Can you work these out from the model? Positions are in its coordinate system, mm. Face numbers are marked on the shaded views. A direction names the side the tool comes from. Give positions to 0.01 mm unless a question says otherwise; leave off trailing zeros. Order: outer loops, then holes, each group sorted by start corner. A loop starts at its lowest first (then second) coordinate and runs counter-clockwise, first axis right, second up. Notation, with made-up numbers: (63, 3.5) - (87, 3.5) arc R19 cw to (87, 7.5) - close; hole circle Ø11 at (30, -6.75). An arc over 180 degrees is marked (long way). Return JSON: item names as keys, results as strings.
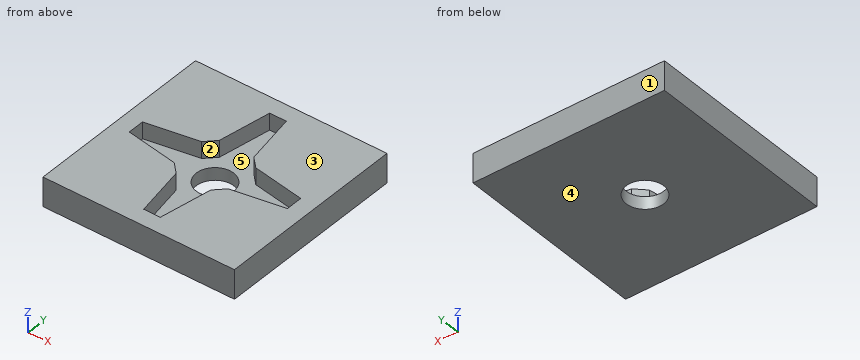
```python
from build123d import *

# Parameters (mm, degrees)
SKETCH1_W           = 46
SKETCH1_H           = 46
BOSS_EXTRUDE1_DEPTH = 7
SKETCH2_W           = 46
SKETCH2_H           = 46
BOSS_EXTRUDE2_DEPTH = 3
SKETCH3_R           = 4.5
CUT_EXTRUDE1_DEPTH  = 3
CUT_EXTRUDE2_DEPTH  = 4


with BuildPart() as part:
    # Sketch1 → Boss-Extrude1 (new body)
    with BuildSketch(Plane.XY):
        Rectangle(SKETCH1_W, SKETCH1_H)
        Polygon((-2, 19), (2, 19), (4.5, 4.5), (19, 2), (19, -2), (4.5, -4.5), (2, -19), (-2, -19), (-4.5, -4.5), (-19, -2), (-19, 2), (-4.5, 4.5), align=None, mode=Mode.SUBTRACT)
    extrude(amount=BOSS_EXTRUDE1_DEPTH)

    # Sketch2 → Boss-Extrude2 (add)
    with BuildSketch(Plane.XY):
        Rectangle(SKETCH2_W, SKETCH2_H)
    extrude(amount=BOSS_EXTRUDE2_DEPTH)

    # Sketch3 → Cut-Extrude1 (cut)
    with BuildSketch(Plane.XY):
        Circle(SKETCH3_R)
    extrude(amount=CUT_EXTRUDE1_DEPTH, mode=Mode.SUBTRACT)

    # Sketch4 → Cut-Extrude2 (cut)
    with BuildSketch(Plane.XY.offset(7)):
        Polygon((-4.155172414, 6.5), (-6.5, 4.155172414), (-6.5, -4.155172414), (-4.155172414, -6.5), (4.155172414, -6.5), (6.5, -4.155172414), (6.5, 4.155172414), (4.155172414, 6.5), align=None)
    extrude(amount=-CUT_EXTRUDE2_DEPTH, mode=Mode.SUBTRACT)


solid = part.part
```
1. Thinking about a two-plate mould opening in Y: for the marked faces 1, 2 and 3, which applies, +Y half, -Y half, draft (parallel to the pull), parting line (faces both ways), or undercut?
Checks:
{"face 1": "+Y half", "face 2": "undercut", "face 3": "draft"}
2. Suppose I cut it at D-D (y = 11). List the corners of the cut face in (x, z) for me.
Checks:
{"outline": "(-23, 0) - (23, 0) - (23, 7) - (3.38, 7) - (3.38, 3) - (-3.38, 3) - (-3.38, 7) - (-23, 7) - close"}
3. On a 3-axis mill with a long thin cutter (end or side, diameter ignored), from which of +Z, -Z, +X, -X, +Y, -Y can I reach the whole of each face in a straight line? I mean the marked faces 4 and 5. Say none if no direction works.
Checks:
{"face 4": "-Z, +X, -X, +Y, -Y", "face 5": "+Z"}
4. If I drill on L1, parallel to Y at x = 0, z = 1.15; L2, parallel to Y at x = -1.5, z = 6.25; L3, parallel to Z at x = -6.5, y = 3, over which ranges is the centre line in solid material (lowest first)? Write a range as [from, to].
Checks:
{"L1": "[-23, -4.5], [4.5, 23]", "L2": "[-23, -19], [19, 23]", "L3": "[0, 3]"}
5. Suppose I cut it at A-A (z = 6.25). List the corners of the cut face in (x, y) for me, plus the area to 3 significant figures.
Checks:
{"outline": "(-23, -23) - (23, -23) - (23, 23) - (-23, 23) - close; hole (-19, -2) - (-6.5, -4.16) - (-4.16, -6.5) - (-2, -19) - (2, -19) - (4.16, -6.5) - (6.5, -4.16) - (19, -2) - (19, 2) - (6.5, 4.16) - (4.16, 6.5) - (2, 19) - (-2, 19) - (-4.16, 6.5) - (-6.5, 4.16) - (-19, 2) - close", "area": "1,650 mm^2"}
6. Suppose I cut it at B-B (y = 0). List the corners of the cut face in (x, z) for me, plus the area to 3 significant figures.
Checks:
{"outline": "(-23, 0) - (-4.5, 0) - (-4.5, 3) - (-19, 3) - (-19, 7) - (-23, 7) - close; (4.5, 0) - (23, 0) - (23, 7) - (19, 7) - (19, 3) - (4.5, 3) - close", "area": "143 mm^2"}
7. For pin 1 Ø14.5 at (x, y) = (0, 0) entering from +Z, with a flat end and sliding along its axis, tell me the tip position at first contact or that it passes through.
Checks:
{"pin 1": "z = 3"}
